Verification items for this drawing (mm, ordinates from the low corner). A direction names the side the tool comes from. Round coordinates to 2 decimals unless told otherwise and drop trailing zeros. Order: outer loops, then holes, each group sorted by start corner. A loop starts at its lowest first (then second) coordinate and runs counter-clockwise, first axis right, second up. Notation, with made-up numbers: (69, 35.25) -> (90, 35.25) arc R30 cw to (90, 57.25) -> close; hole circle Ø11 at (7.5, 51.5). An arc over 180 degrees is marked (long way). Put each result on its own line as item: value.
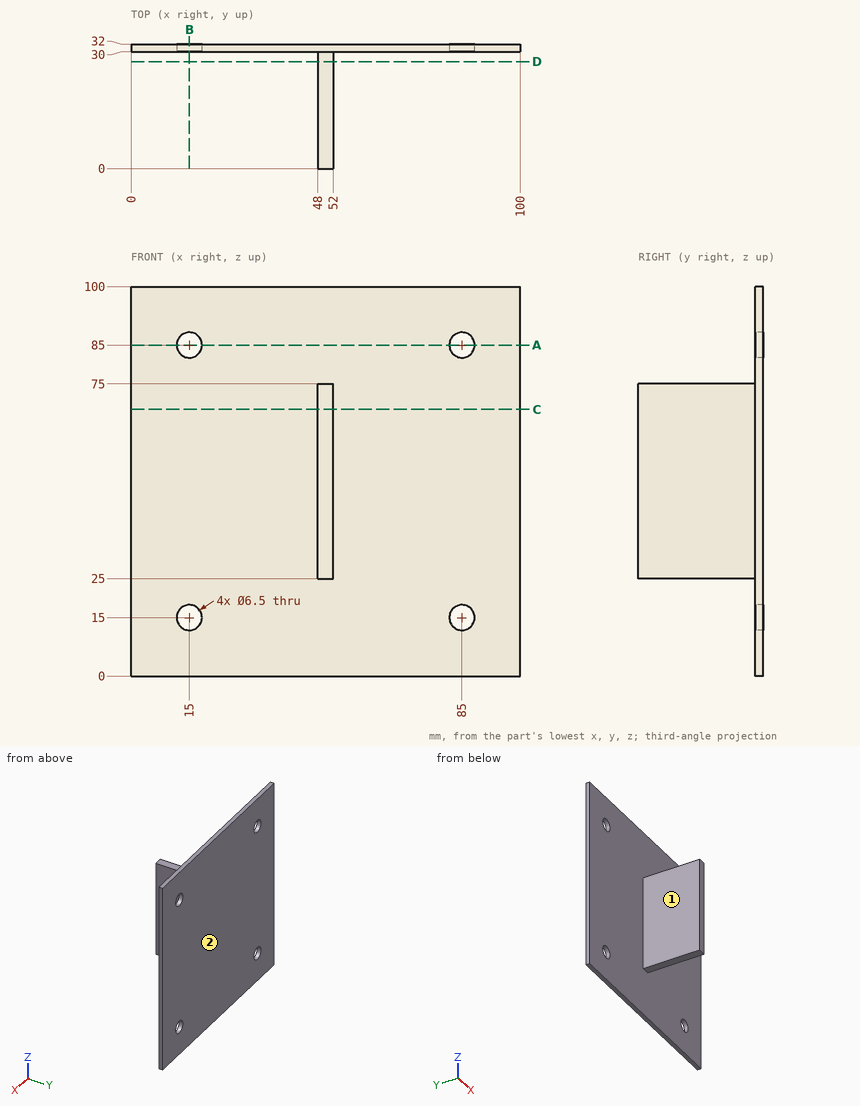
Item 1: Gauge pin test, flat ends, axial feed: pin 1 Ø6 at (x, y) = (44, 18.5) entering from -Z; pin 2 Ø10 at (y, z) = (16, 79) entering from -X; pin 3 Ø4.5 at (x, y) = (50.5, 18.5) entering from -Z; pin 4 Ø7.5 at (x, z) = (15, 85) entering from +Y. Record the tip position at first contact, or that the pin passes through.
Check sheet entries:
pin 1: passes through
pin 2: stops at x = 48
pin 3: stops at z = 25
pin 4: stops at y = 32
Item 2: Section check B-B on x = 15. Record the boundary of the cut face in (y, z), then the cut area to 3 significant figures.
Check sheet entries:
outline: (30, 0) -> (32, 0) -> (32, 11.75) -> (30, 11.75) -> close; (30, 18.25) -> (32, 18.25) -> (32, 81.75) -> (30, 81.75) -> close; (30, 88.25) -> (32, 88.25) -> (32, 100) -> (30, 100) -> close
area: 174 mm^2
Item 3: Section check C-C on z = 68.5. Record the boundary of the cut face in (x, y).
Check sheet entries:
outline: (0, 30) -> (48, 30) -> (48, 0) -> (52, 0) -> (52, 30) -> (100, 30) -> (100, 32) -> (0, 32) -> close
Item 4: Tool access check on the marked faces 1 and 2. Record the directions out of +Z, -Z, +X, -X, +Y, -Y that give a thin tool (end or side, any length) a straight path to the whole face; none if there is none.
Check sheet entries:
face 1: +Z, -Z, -X, -Y
face 2: +Z, -Z, +X, -X, +Y
Item 5: Material ranges on L1, parallel to Z at x = 85, y = 31.65; L2, parallel to Y at x = 85.5, z = 56.5; L3, parallel to X at y = 24, z = 32.5, recorded low to high. Write a range as [from, to].
Check sheet entries:
L1: z = [0, 11.75], [18.25, 81.75], [88.25, 100]
L2: y = [30, 32]
L3: x = [48, 52]
Item 6: Section check D-D on y = 27.5. Record the boundary of the cut face in (x, z).
Check sheet entries:
outline: (48, 25) -> (52, 25) -> (52, 75) -> (48, 75) -> close
Item 7: Section check A-A on z = 85. Record the boundary of the cut face in (x, y), then the cut area to 3 significant figures.
Check sheet entries:
outline: (0, 30) -> (11.75, 30) -> (11.75, 32) -> (0, 32) -> close; (18.25, 30) -> (81.75, 30) -> (81.75, 32) -> (18.25, 32) -> close; (88.25, 30) -> (100, 30) -> (100, 32) -> (88.25, 32) -> close
area: 174 mm^2
